Build history of the part. All positions in model axes, mm. A direction names the side the tool comes from. Give positions to 0.01 mm unless a question says otherwise; leave off trailing zeros. Write each loop counter-clockwise with the first axis right and the second up, starting at its lowest first coordinate (ties: lowest second). Pieces come first, ordered by that corner, then holes.
from build123d import *

# Parameters (mm, degrees)
SKETCH1_R           = 1.5
BOSS_EXTRUDE1_DEPTH = 2.159
CUT_EXTRUDE1_DEPTH  = 3.159


with BuildPart() as part:
    # Sketch1 → Boss-Extrude1 (new body)
    with BuildSketch(Plane.XY):
        with BuildLine():
            Line((-9.906, 12.319), (8.872225801, 12.319))
            ThreePointArc((8.872225801, 12.319), (15.338010208, 9.640784407), (18.016225801, 3.175))
            Line((18.016225801, 3.175), (18.016225801, -3.175))
            ThreePointArc((18.016225801, -3.175), (15.338010208, -9.640784407), (8.872225801, -12.319))
            Line((8.872225801, -12.319), (-9.906, -12.319))
            ThreePointArc((-9.906, -12.319), (-16.371784407, -9.640784407), (-19.05, -3.175))
            Line((-19.05, -3.175), (-19.05, 3.175))
            ThreePointArc((-19.05, 3.175), (-16.371784407, 9.640784407), (-9.906, 12.319))
        make_face()
        with Locations((-12.7, 7.874)):
            Circle(SKETCH1_R, mode=Mode.SUBTRACT)
        with Locations((-12.7, -7.874)):
            Circle(SKETCH1_R, mode=Mode.SUBTRACT)
        with Locations((12.7, 7.874)):
            Circle(SKETCH1_R, mode=Mode.SUBTRACT)
        with Locations((12.7, -7.874)):
            Circle(SKETCH1_R, mode=Mode.SUBTRACT)
    extrude(amount=BOSS_EXTRUDE1_DEPTH)

    # Sketch4 → Cut-Extrude1 (cut, through all)
    with BuildSketch(Plane.XY.offset(2.159)):
        with BuildLine():
            Line((-6.755, 9.144), (5.721225801, 9.144))
            ThreePointArc((5.721225801, 9.144), (6.991225801, 7.874), (5.721225801, 6.604))
            Line((5.721225801, 6.604), (-6.755, 6.604))
            ThreePointArc((-6.755, 6.604), (-8.025, 7.874), (-6.755, 9.144))
        make_face()
        with BuildLine():
            Line((-12.7, 3.894666667), (11.666225801, 3.894666667))
            ThreePointArc((11.666225801, 3.894666667), (12.936225801, 2.624666667), (11.666225801, 1.354666667))
            Line((11.666225801, 1.354666667), (-12.7, 1.354666667))
            ThreePointArc((-12.7, 1.354666667), (-13.97, 2.624666667), (-12.7, 3.894666667))
        make_face()
        with BuildLine():
            Line((-12.7, -1.354666667), (11.666225801, -1.354666667))
            ThreePointArc((11.666225801, -1.354666667), (12.936225801, -2.624666667), (11.666225801, -3.894666667))
            Line((11.666225801, -3.894666667), (-12.7, -3.894666667))
            ThreePointArc((-12.7, -3.894666667), (-13.97, -2.624666667), (-12.7, -1.354666667))
        make_face()
        with BuildLine():
            Line((-6.755, -6.604), (5.721225801, -6.604))
            ThreePointArc((5.721225801, -6.604), (6.991225801, -7.874), (5.721225801, -9.144))
            Line((5.721225801, -9.144), (-6.755, -9.144))
            ThreePointArc((-6.755, -9.144), (-8.025, -7.874), (-6.755, -6.604))
        make_face()
    extrude(amount=-CUT_EXTRUDE1_DEPTH, mode=Mode.SUBTRACT)


solid = part.part
1. Saw through at A-A on x = 10. Give the cut face in (y, z), plus the area to 3 significant figures.
2. Saw through at D-D on y = -2.5. Give the cut face in (x, z).
3. Saw through at B-B on y = 7.25. Give the cut face in (x, z).
4. Saw through at C-C on z = 0.6. Count the separate pieces of the cut face and the enclosed holes in it, plus the area to 3 significant figures.
5. Mould opens along Y. For faces 1 (the face through (0, -12.319, 1)), 2 (the face through (-19.05, 0, 1)), 3 (the face through (-8.025, -7.902, 1.095)) say: pulls with the +Y half, pulls with the -Y half, needs draft (parallel to the pull), parting line crosses it, or undercut.
6. 3-axis set-ups, long thin cutter, end or side, ignore diameter. For faces 4 (the face through (15.27, 9.71, 1.06)), 5 (the face through (-1, 3.895, 1)): which of +Z, -Z, +X, -X, +Y, -Y reach the whole face in a straight line?
7. Drill centre lines: line 1 along Y through (x, z) = (-4, 1.2); line 2 along Y through (x, z) = (7.5, 0.3); line 3 along X through (y, z) = (-6.5, 1.6). Where is each one in solid material? Low to high.
Outcome:
1. outline: (-12.25, 0) - (-3.89, 0) - (-3.89, 2.16) - (-12.25, 2.16) - close; (-1.35, 0) - (1.35, 0) - (1.35, 2.16) - (-1.35, 2.16) - close; (3.89, 0) - (12.25, 0) - (12.25, 2.16) - (3.89, 2.16) - close
1. area: 41.9 mm2
2. outline: (-19.05, 0) - (-13.96, 0) - (-13.96, 2.16) - (-19.05, 2.16) - close; (12.93, 0) - (18.02, 0) - (18.02, 2.16) - (12.93, 2.16) - close
3. outline: (-18.09, 0) - (-14.06, 0) - (-14.06, 2.16) - (-18.09, 2.16) - close; (-11.34, 0) - (-7.86, 0) - (-7.86, 2.16) - (-11.34, 2.16) - close; (6.83, 0) - (11.34, 0) - (11.34, 2.16) - (6.83, 2.16) - close; (14.06, 0) - (17.06, 0) - (17.06, 2.16) - (14.06, 2.16) - close
4. separate pieces: 1
4. enclosed holes: 8
4. area: 606 mm2
5. face 1: pulls with the -Y half
5. face 2: needs draft
5. face 3: undercut
6. face 4: +Z, -Z, +X, +Y
6. face 5: +Z, -Z
7. line 1: y = -12.32 to -9.14, -6.6 to -3.89, -1.35 to 1.35, 3.89 to 6.6, 9.14 to 12.32
7. line 2: y = -12.32 to -3.89, -1.35 to 1.35, 3.89 to 12.32
7. line 3: x = -18.42 to -13.3, -12.1 to 12.1, 13.3 to 17.39
